Input: part model. Units: mm. Frame: model coordinates. A direction names the side the tool comes from. Coordinates: 2 decimals unless noted, no trailing zeros. Write each loop counter-clockwise with the first axis right and the second up, starting at its lowest first coordinate (ties: lowest second). Pieces come first, ordered by that corner, then holes. Notation, with made-up numbers: M 1,-14 L 10,-14 A21 cw 10,1 Z; hole C 28.5,3 d8. An arc over 180 degrees is marked long. Use one line per item in the form item = value.
from build123d import *

# Parameters (mm, degrees)
SKETCH1_R           = 1
SKETCH1_R_2         = 0.910218414
SKETCH1_R_3         = 0.906034418
BOSS_EXTRUDE1_DEPTH = 2


with BuildPart() as part:
    # Sketch1 → Boss-Extrude1 (new body)
    with BuildSketch(Plane.XY):
        Polygon((-20.265114669, -14.781853255), (0, -14.781853255), (2.578230219, -12.031741021), (9.974883423, -12.031741021), (11.921608737, -14.781853255), (11.921608737, -20.387219314), (16.856252033, -20.387219314), (19.428429521, -14.668134436), (16.109635951, -5.526454973), (13.99339942, -5.01215501), (7.32119149, 13.172265413), (9.371469902, 17.730938487), (5.533408169, 26.134970212), (7.143643167, 29.715232721), (4.143999648, 36.283417669), (0.771614698, 37.274543445), (0.269863196, 36.158928585), (-5.511384257, 38.825843561), (-6.442002374, 40.863576334), (-9.378393977, 42.218146745), (-12.56174706, 40.764331952), (-13.563489591, 36.865253111), (-9.034751731, 32.619561367), (-8.044765523, 30.451832945), (-10.970070519, 16.504069812), (-13.563489591, 15.919840508), (-16.715889982, 0.889293603), (-15.139689787, -0.58839408), (-16.175363684, -5.526454973), (-22.571570479, -8.447557289), (-22.571570479, -12.031741021), align=None)
        with Locations((-18.892731675, -12.928934576)):
            Circle(SKETCH1_R, mode=Mode.SUBTRACT)
        with Locations((14.921608737, -17.281853255)):
            Circle(SKETCH1_R, mode=Mode.SUBTRACT)
        with Locations((-2.044247077, -6.842384565)):
            Circle(SKETCH1_R, mode=Mode.SUBTRACT)
        with Locations((5.01567612, 23.865741995)):
            Circle(SKETCH1_R_2, mode=Mode.SUBTRACT)
        with Locations((-4.254696048, 27.615435298)):
            Circle(SKETCH1_R_3, mode=Mode.SUBTRACT)
        Polygon((2.128672216, -1.518848285), (-6.871327784, -1.518848285), (-9.371327784, 1.510447631), (-8.371327784, 6.908565954), (-6.871327784, 8.46349525), (-5.519746073, 12.22825254), (-6.7697323, 13.478238768), (-6.7697323, 17.009479478), (-2.371327784, 21.568951505), (2.027076733, 17.009479478), (2.681238146, 13.478238768), (1.431251918, 12.22825254), (2.128672216, 8.46349525), (3.628672216, 6.908565954), (4.628672216, 1.510447631), align=None, mode=Mode.SUBTRACT)
    extrude(amount=BOSS_EXTRUDE1_DEPTH)


solid = part.part
(1) Line query: probe 1 along Y at (x, z) = (-2, 1.1); probe 2 along Y at (x, z) = (-4, 1.4); probe 3 along X at (y, z) = (11, 0.75). Output: solid intervals per line, ascending.
Computed:
probe_1 = -14.78 to -7.84, -5.84 to -1.52, 21.18 to 37.21
probe_2 = -14.78 to -1.52, 19.88 to 26.75, 28.48 to 38.13
probe_3 = -14.6 to -5.96, 1.66 to 8.12
(2) Set-up query: faces 1 (the flat face through (1.27, -13.43, 0.99)), 2 (the flat face through (2.065, 12.862, 0.986)), 3 (the flat face through (-12.249, 16.216, 0.986)). Return all of +Z, -Z, +X, -X, +Y, -Y with unobstructed straight access to the full face (end or side cutting, diameter ignored); none if empty.
Computed:
face_1 = +Z, -Z, -Y
face_2 = +Z, -Z
face_3 = +Z, -Z, -X
(3) Section query A-A on y = 10. Return the cut outline in (x, z).
Computed:
outline = M -14.81,0 L -6.32,0 L -6.32,2 L -14.81,2 Z; M 1.84,0 L 8.49,0 L 8.49,2 L 1.84,2 Z
(4) Section query C-C on z = 1.45. State how many separate pieces and enclosed holes the cut face has, plus the area to 3 significant figures.
Computed:
separate_pieces = 1
enclosed_holes = 6
area = 1,080 mm^2
(5) Pull-direction query (X, two-part tool) for faces 4 (the flat face through (-2.58, 37.474, 0.986)), 5 (the flat face through (17.79, -10.16, 0.99)), 6 (the flat face through (-13.056, 38.842, 0.986)); classes: pulls with the +X half, pulls with the -X half, needs draft (parallel to the pull), parting line crosses it, or undercut.
Computed:
face_4 = undercut
face_5 = pulls with the +X half
face_6 = pulls with the -X half
(6) First-contact query: pin 1 Ø0.6 at (y, z) = (-17.5, 1) entering from -X; pin 2 Ø1 at (x, z) = (0, 0.5) entering from +Y; pin 3 Ø1 at (x, z) = (-13.5, 1.5) entering from -Y. Flat tips, straight axial feed; report the tip coordinate or a pass-through.
Computed:
pin_1 = 11.92
pin_2 = 36.67
pin_3 = -14.78
(7) Section query B-B on x = 8.5. Return the cut outline in (y, z).
Computed:
outline = M -12.03,0 L 9.96,0 L 9.96,2 L -12.03,2 Z; M 15.79,0 L 19.64,0 L 19.64,2 L 15.79,2 Z
